Geometry: final body of the model. Coordinates: model frame, mm. A direction names the side the tool comes from. Coordinates: 2 decimals unless noted, no trailing zeros. Write each loop counter-clockwise with the first axis right and the second up, starting at its lowest first coordinate (ties: lowest second). Pieces come first, ordered by that corner, then holes. Notation, with made-up numbers: (21, 35) -> (37, 35) arc R24 ccw to (37, 74) -> close; hole circle Ø6 at (84.5, 13). An arc over 180 degrees is marked (long way). Answer as a JSON object with one key per item and string values. Group by question number.
```python
from build123d import *

# Parameters (mm, degrees)
SKETCH1_W                = 14.2748
SKETCH1_H                = 7.874
BOSS_EXTRUDE1_DEPTH      = 3.937
BOSS_EXTRUDE1_DEPTH_BACK = 3.937
SKETCH2_W                = 9.4996
SKETCH2_H                = 3.556
CUT_EXTRUDE1_DEPTH       = 3.937
CUT_EXTRUDE1_DEPTH_BACK  = 3.937
SKETCH4_W                = 0.2032
SKETCH4_H                = 1.26365
SKETCH5_W                = 7.874
SKETCH5_H                = 1.61925


with BuildPart() as part:
    # Sketch1 → Boss-Extrude1 (new body, two sides)
    with BuildSketch(Plane.XY) as boss_extrude1_sk:
        with Locations((3.9878, 0)):
            Rectangle(SKETCH1_W, SKETCH1_H)
    extrude(amount=BOSS_EXTRUDE1_DEPTH)
    extrude(boss_extrude1_sk.sketch, amount=-BOSS_EXTRUDE1_DEPTH_BACK)

    # Sketch2 → Cut-Extrude1 (cut, two sides)
    with BuildSketch(Plane(origin=(0, 0, 0), x_dir=(1, 0, 0), z_dir=(0, 1, 0))) as cut_extrude1_sk:
        with Locations((1.6002, 0)):
            Rectangle(SKETCH2_W, SKETCH2_H)
    extrude(amount=CUT_EXTRUDE1_DEPTH, mode=Mode.SUBTRACT)
    extrude(cut_extrude1_sk.sketch, amount=-CUT_EXTRUDE1_DEPTH_BACK, mode=Mode.SUBTRACT)

    # Sketch3 → Cut-Revolve1 (revolve, cut)
    with BuildSketch(Plane.XY):
        Polygon((6.5532, 0), (6.5532, 1.24333), (10.78103, 1.24333), (11.1252, 1.5875), (11.1252, 0), align=None)
    revolve(axis=Axis((11.1252, 0, 0), (-1, 0, 0)), mode=Mode.SUBTRACT)

    # Sketch4 → Cut-Revolve2 (revolve, cut)
    with BuildSketch(Plane.XY):
        with Locations((6.4516, 0.631825)):
            Rectangle(SKETCH4_W, SKETCH4_H)
    revolve(axis=Axis((6.5532, 0, 0), (-1, 0, 0)), mode=Mode.SUBTRACT)

    # Sketch5 → Cut-Revolve3 (revolve, cut)
    with BuildSketch(Plane(origin=(0, 0, 0), x_dir=(0, 0, -1), z_dir=(1, 0, 0))):
        with Locations((0, 0.809625)):
            Rectangle(SKETCH5_W, SKETCH5_H)
    revolve(axis=Axis((0, 0, -3.937), (0, 0, 1)), mode=Mode.SUBTRACT)

    # Sketch6 → Cut-Revolve4 (revolve, cut)
    with BuildSketch(Plane.XY):
        with BuildLine():
            Line((11.1252, 0), (11.1252, 3.937))
            ThreePointArc((11.1252, 3.937), (10.164844056, 6.105270359), (8.5852, 7.874))
            Line((8.5852, 7.874), (15.0622, 7.874))
            Line((15.0622, 7.874), (15.0622, 0))
            Line((15.0622, 0), (11.1252, 0))
        make_face()
    revolve(axis=Axis((15.0622, 0, 0), (-1, 0, 0)), mode=Mode.SUBTRACT)

    # Sketch7 → Cut-Revolve5 (revolve, cut)
    with BuildSketch(Plane.XY):
        with BuildLine():
            Line((-7.0866, 0), (-7.0866, 7.874))
            Line((-7.0866, 7.874), (-0.6096, 7.874))
            ThreePointArc((-0.6096, 7.874), (-2.189244056, 6.105270359), (-3.1496, 3.937))
            Line((-3.1496, 3.937), (-3.1496, 0))
            Line((-3.1496, 0), (-7.0866, 0))
        make_face()
    revolve(axis=Axis((-3.1496, 0, 0), (-1, 0, 0)), mode=Mode.SUBTRACT)


solid = part.part
```
Item 1: Mould query, pull axis Y, two halves, no side actions, for faces 3 (the flat face through (11.125, 2, 0)), 4 (the flat face through (6, -3.937, 2)), 5 (the cylindrical face through (8.697, -0.162, -1.233)). Classes: +Y half, -Y half, draft (parallel to the pull), parting line (faces both ways), or undercut.
Item 2: Section B-B on x = 0. Output: boundary loops of the cut face in (y, z), then the cut area to 3 significant figures.
Item 3: Ray query, L1, parallel to Z at x = 2, y = 1; L2, parallel to X at y = 0, z = 2.8; L3, parallel to Y at x = 0, z = 2.85. Return the intervals inside material, ascending. Write a range as [from, to].
Item 4: Section C-C on x = 10. Output: boundary loops of the cut face in (y, z), then the cut area to 3 significant figures.
Item 5: Set-up query: faces 1 (the flat face through (6, 3.937, 2)), 2 (the flat face through (6.35, 1, 1)). Return all of +Z, -Z, +X, -X, +Y, -Y with unobstructed straight access to the full face (end or side cutting, diameter ignored); none if empty.
Item 6: Section D-D on y = -0.25. Give the number of separate pieces and of enclosed holes in the cut face, then the cut area to 3 significant figures.
Item 7: Contact query for flat-ended pins moving along their axis: pin 1 (1.5 mm diameter, centred on y = 0, z = 0, fed in from +X); pin 2 (4 mm diameter, centred on y = -1.5, z = 1, fed in from -X). Output: stop coordinate, or through.
Item 8: Section A-A on x = 4. Output: boundary loops of the cut face in (y, z).
Answer sheet:
{
 "1": {"face 3": "draft", "face 4": "-Y half", "face 5": "undercut"},
 "2": {"outline": "(-3.94, -3.94) -> (-1.62, -3.94) -> (-1.62, -1.78) -> (-3.94, -1.78) -> close; (-3.94, 1.78) -> (-1.62, 1.78) -> (-1.62, 3.94) -> (-3.94, 3.94) -> close; (1.62, -3.94) -> (3.94, -3.94) -> (3.94, -1.78) -> (1.62, -1.78) -> close; (1.62, 1.78) -> (3.94, 1.78) -> (3.94, 3.94) -> (1.62, 3.94) -> close", "area": "20.0 mm^2"},
 "3": {"L1": "z = [-3.94, -1.78], [1.78, 3.94]", "L2": "x = [-3.15, -1.62], [1.62, 11.13]", "L3": "y = [-3.94, -1.62], [1.62, 3.94]"},
 "4": {"outline": "(-3.94, -3.94) -> (3.94, -3.94) -> (3.94, 3.94) -> (-3.94, 3.94) -> close; hole circle Ø2.49 at (0, 0)", "area": "57.1 mm^2"},
 "5": {"face 1": "+Z, -Z, +X, -X, +Y", "face 2": "-X, +Y, -Y"},
 "6": {"separate pieces": "4", "enclosed holes": "0", "area": "53.0 mm^2"},
 "7": {"pin 1": "passes through", "pin 2": "stops at x = -3.15"},
 "8": {"outline": "(-3.94, -3.94) -> (3.94, -3.94) -> (3.94, -1.78) -> (-3.94, -1.78) -> close; (-3.94, 1.78) -> (3.94, 1.78) -> (3.94, 3.94) -> (-3.94, 3.94) -> close"}
}
